from build123d import *

# Parameters (mm, degrees)
AUFSATZ_LINEAR_AUSTRAGEN1_DEPTH = 20
SKIZZE2_W                       = 25
SKIZZE2_H                       = 3.4
SCHNITT_LINEAR_AUSTRAGEN1_DEPTH = 84.234848471
VERRUNDUNG1_R                   = 3
VERRUNDUNG2_R                   = 6
SCHNITT_LINEAR_AUSTRAGEN2_DEPTH = 80.063518768


with BuildPart() as part:
    # Skizze1 → Aufsatz-Linear austragen1 (new body)
    with BuildSketch(Plane(origin=(0, 0, 0), x_dir=(1, 0, 0), z_dir=(0, 1, 0))):
        Polygon((0, 0), (0, 35), (60.2, 35), (60.2, 0), (65.2, 0), (65.2, 40), (-5, 40), (-5, 0), align=None)
    extrude(amount=AUFSATZ_LINEAR_AUSTRAGEN1_DEPTH)

    # Skizze2 → Schnitt-Linear austragen1 (cut, through all)
    with BuildSketch(Plane.ZY.offset(5)):
        with Locations((-14.5, 10)):
            Rectangle(SKIZZE2_W, SKIZZE2_H)
    extrude(amount=-SCHNITT_LINEAR_AUSTRAGEN1_DEPTH, mode=Mode.SUBTRACT)

    # Verrundung1
    verrundung1_edges = [part.edges().sort_by_distance(p)[0] for p in [
        (60.2, 10, -35),
        (0, 10, -35),
    ]]
    fillet(verrundung1_edges, radius=VERRUNDUNG1_R)

    # Verrundung2
    verrundung2_edges = [part.edges().sort_by_distance(p)[0] for p in [
        (-5, 10, -40),
        (65.2, 10, -40),
    ]]
    fillet(verrundung2_edges, radius=VERRUNDUNG2_R)

    # Skizze3 → Schnitt-Linear austragen2 (cut, through all)
    with BuildSketch(Plane(origin=(0, 0, -40), x_dir=(-1, 0, 0), z_dir=(0, 0, -1))):
        Polygon((-45.1, 5), (-15.1, 5), (-10.1, 0), (-50.1, 0), align=None)
    extrude(amount=-SCHNITT_LINEAR_AUSTRAGEN2_DEPTH, mode=Mode.SUBTRACT)


solid = part.part
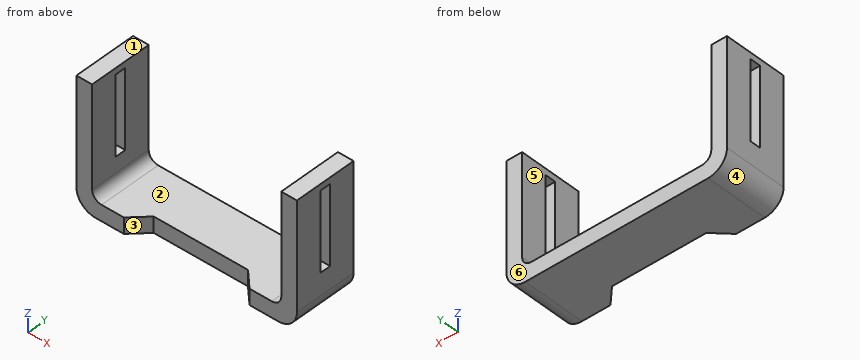
Work out the finished part from the listing and answer in its coordinate system (mm). Face numbers are marked on the shaded views. A direction names the side the tool comes from. Coordinates: 2 decimals unless noted, no trailing zeros. Write each loop counter-clockwise with the first axis right and the second up, starting at its lowest first coordinate (ties: lowest second). Pieces come first, ordered by that corner, then holes. Notation, with made-up numbers: M -11.5,13.5 L 39.5,13.5 A33 ccw 39.5,41.5 Z; hole C 46,24 d6. An arc over 180 degrees is marked long. Answer as CSV lines item,"result". Start each with the question number.
Item 1: Determine the mould class of the marked faces 4, 5 and 6 for opening direction X: released by +X, released by -X, zero draft, split by the parting line, or undercut.
Item 2: A tool of negligible diameter and unlimited length cuts with its end or side. For the marked faces 1, 2 and 3, from which of +Z, -Z, +X, -X, +Y, -Y can it reach the whole face along a straight path? Write none if from no direction.
Item 3: Section D-D on z = -18 is taken. Write down the section's boundary in (x, y), and give its area (3 significant figures).
Item 4: Section C-C on z = -29.5 is taken. Write down the section's boundary in (x, y).
Item 5: Section A-A on y = 10 is taken. Write down the section's boundary in (x, z).
Item 6: Flat-ended cylindrical pins translate along their axes: P1, Ø10, axis at y = 9, z = -16.5, coming from the +X side; P2, Ø8, axis at x = 41.5, y = 16, coming from the +Z side; P3, Ø2.5, axis at x = 36, z = -36.5, coming from the -Y side; P4, Ø3.5, axis at x = -1.5, y = 11, coming from the -Z side. Find the tip coordinate at first contact, or state that the pin passes through.
Item 7: Section B-B on y = 3.75 is taken. Write down the section's boundary in (x, z), and give its area (3 significant figures).
Item 8: Consider L1, parallel to X at y = 18.75, z = -22; L2, parallel to Z at x = 4, y = 17.5; L3, parallel to Y at x = 62, z = -6. Determine where each line is inside the solid, lowest interval first.
Checks:
1,face 4,"released by -X"
1,face 5,"undercut"
1,face 6,"zero draft"
2,face 1,"+Z, +X, -X, +Y, -Y"
2,face 2,"+Z, +Y, -Y"
2,face 3,"+Z, -Z, -Y"
3,outline,"M -5,0 L 0,0 L 0,8.3 L -5,8.3 Z; M -5,11.7 L 0,11.7 L 0,20 L -5,20 Z; M 60.2,0 L 65.2,0 L 65.2,8.3 L 60.2,8.3 Z; M 60.2,11.7 L 65.2,11.7 L 65.2,20 L 60.2,20 Z"
3,area,"166 mm²"
4,outline,"M -5,0 L 0,0 L 0,20 L -5,20 Z; M 60.2,0 L 65.2,0 L 65.2,20 L 60.2,20 Z"
5,outline,"M -5,-34 A6 ccw 1,-40 L 59.2,-40 A6 ccw 65.2,-34 L 65.2,-27 L 60.2,-27 L 60.2,-32 A3 cw 57.2,-35 L 3,-35 A3 cw 0,-32 L 0,-27 L -5,-27 Z; M -5,-2 L 0,-2 L 0,0 L -5,0 Z; M 60.2,-2 L 65.2,-2 L 65.2,0 L 60.2,0 Z"
6,P1,"stops at x = 65.2"
6,P2,"stops at z = -35"
6,P3,"stops at y = 5"
6,P4,"stops at z = -39.95"
7,outline,"M -5,-34 A6 ccw 1,-40 L 13.85,-40 L 13.85,-35 L 3,-35 A3 cw 0,-32 L 0,0 L -5,0 Z; M 46.35,-40 L 59.2,-40 A6 ccw 65.2,-34 L 65.2,0 L 60.2,0 L 60.2,-32 A3 cw 57.2,-35 L 46.35,-35 Z"
7,area,"527 mm²"
8,L1,"x = -5 to 0, 60.2 to 65.2"
8,L2,"z = -40 to -35"
8,L3,"y = 0 to 8.3, 11.7 to 20"
